For this review, take the finished solid that the model builds, in its own axes (mm). Face numbers are marked on the shaded views. A direction names the side the tool comes from. Coordinates: 2 decimals unless noted, no trailing zeros. Loops run counter-clockwise (first coordinate to the right, second up) from the corner with the lowest first, then second, coordinate; pieces in that order, holes last. Notation, with made-up numbers: M 20,-12 L 44,-12 A21 ccw 44,9 Z; hole C 58.25,61.5 d9. An arc over 180 degrees is marked long. Put each result on its own line as item: value.
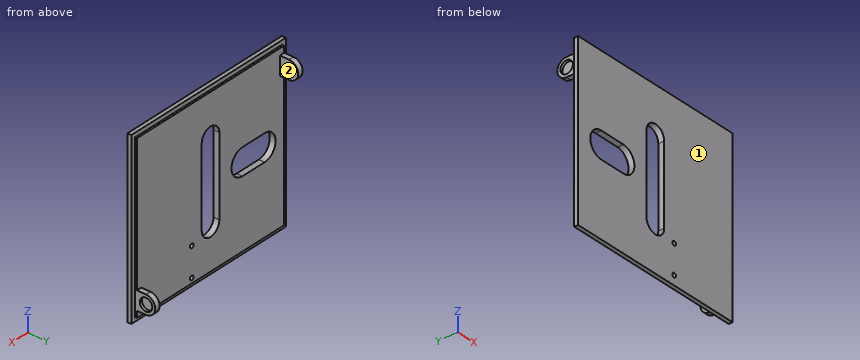
```python
from build123d import *

# Parameters (mm, degrees)
SKETCH1_W                       = 140
SKETCH1_H                       = 130
BOSS_EXTRUDE1_DEPTH             = 3
SKETCH2_W                       = 133.6
SKETCH2_H                       = 123.6
BOSS_EXTRUDE2_DEPTH             = 1.5
SKETCH5_W                       = 4
SKETCH5_H                       = 14
BOSS_EXTRUDE3_DEPTH             = 14
SKETCH6_R                       = 4.775
CUT_EXTRUDE3_DEPTH              = 2
FILLET1_RADIUS                  = 7
FILLET1_LENGTH                  = 4
CIRPATTERN2_COUNT               = 2
FILLET1_OF_CIRPATTERN2_2_RADIUS = 7
FILLET1_OF_CIRPATTERN2_2_LENGTH = 4
CUT_EXTRUDE4_DEPTH              = 97.545326143
CUT_EXTRUDE5_DEPTH              = 98.29979445
SKETCH9_R                       = 1.6
CUT_EXTRUDE6_DEPTH              = 98.29979445


with BuildPart() as part:
    # Sketch1 → Boss-Extrude1 (new body)
    with BuildSketch(Plane(origin=(0, 0, 0), x_dir=(1, 0, 0), z_dir=(0, 1, 0))):
        Rectangle(SKETCH1_W, SKETCH1_H)
    extrude(amount=BOSS_EXTRUDE1_DEPTH)

    # Sketch2 → Boss-Extrude2 (add)
    with BuildSketch(Plane(origin=(0, 3, 0), x_dir=(1, 0, 0), z_dir=(0, 1, 0))):
        Rectangle(SKETCH2_W, SKETCH2_H)
    extrude(amount=BOSS_EXTRUDE2_DEPTH)

    # Sketch5 → Boss-Extrude3 (add)
    with BuildSketch(Plane(origin=(0, 4.5, 0), x_dir=(1, 0, 0), z_dir=(0, 1, 0))):
        with Locations((-64.8, -49.8)):
            Rectangle(SKETCH5_W, SKETCH5_H)
    boss_extrude3 = extrude(amount=BOSS_EXTRUDE3_DEPTH)

    # Sketch6 → Cut-Extrude3 (cut)
    with BuildSketch(Plane.ZY.offset(66.8)):
        with Locations((49.8, 11.5)):
            Circle(SKETCH6_R)
    cut_extrude3 = extrude(amount=-CUT_EXTRUDE3_DEPTH, mode=Mode.SUBTRACT)

    # Fillet1: full round fillet: the end face becomes a half cylinder, R = half its width
    fillet1_face = Plane((-64.8, 18.5, 49.8), x_dir=(1, 0, 0), z_dir=(0, 1, 0))  # on the end face: x along it, z out of the body
    fillet1_slab = fillet1_face.offset(-FILLET1_RADIUS / 2) * Box(FILLET1_LENGTH, 2 * FILLET1_RADIUS, FILLET1_RADIUS, mode=Mode.PRIVATE)  # the body's end, R deep
    fillet1_round = Plane((-64.8, 11.5, 49.8), x_dir=(0, 1, 0), z_dir=(1, 0, 0)) * Cylinder(FILLET1_RADIUS, FILLET1_LENGTH, mode=Mode.PRIVATE)  # its axis R under the face
    add(fillet1_slab - fillet1_round, mode=Mode.SUBTRACT)

    # CirPattern2: Boss-Extrude3, Cut-Extrude3 ×2 about axis
    cirpattern2_axis = Axis((0, 0, 0), (0, 1, 0))
    add([boss_extrude3.rotate(cirpattern2_axis, i * 360 / CIRPATTERN2_COUNT) for i in range(1, CIRPATTERN2_COUNT)])
    add([cut_extrude3.rotate(cirpattern2_axis, i * 360 / CIRPATTERN2_COUNT) for i in range(1, CIRPATTERN2_COUNT)], mode=Mode.SUBTRACT)

    # Fillet1 of CirPattern2 2: full round fillet: the end face becomes a half cylinder, R = half its width
    fillet1_of_cirpattern2_2_face = Plane((64.8, 18.5, -49.8), x_dir=(-1, 0, 0), z_dir=(0, 1, 0))  # on the end face: x along it, z out of the body
    fillet1_of_cirpattern2_2_slab = fillet1_of_cirpattern2_2_face.offset(-FILLET1_OF_CIRPATTERN2_2_RADIUS / 2) * Box(FILLET1_OF_CIRPATTERN2_2_LENGTH, 2 * FILLET1_OF_CIRPATTERN2_2_RADIUS, FILLET1_OF_CIRPATTERN2_2_RADIUS, mode=Mode.PRIVATE)  # the body's end, R deep
    fillet1_of_cirpattern2_2_round = Plane((64.8, 11.5, -49.8), x_dir=(0, 1, 0), z_dir=(-1, 0, 0)) * Cylinder(FILLET1_OF_CIRPATTERN2_2_RADIUS, FILLET1_OF_CIRPATTERN2_2_LENGTH, mode=Mode.PRIVATE)  # its axis R under the face
    add(fillet1_of_cirpattern2_2_slab - fillet1_of_cirpattern2_2_round, mode=Mode.SUBTRACT)

    # Sketch7 → Cut-Extrude4 (cut, through all)
    with BuildSketch(Plane(origin=(0, 4.5, 0), x_dir=(1, 0, 0), z_dir=(0, 1, 0))):
        with BuildLine():
            Line((-8, -30), (-8, 30))
            ThreePointArc((-8, 30), (0, 38), (8, 30))
            Line((8, 30), (8, -30))
            ThreePointArc((8, -30), (0, -38), (-8, -30))
        make_face()
    extrude(amount=-CUT_EXTRUDE4_DEPTH, mode=Mode.SUBTRACT)

    # Sketch8 → Cut-Extrude5 (cut, through all)
    with BuildSketch(Plane.XZ):
        with BuildLine():
            Line((-49, 10), (-29, 10))
            ThreePointArc((-29, 10), (-19, 0), (-29, -10))
            Line((-29, -10), (-49, -10))
            ThreePointArc((-49, -10), (-59, 0), (-49, 10))
        make_face()
    extrude(amount=-CUT_EXTRUDE5_DEPTH, mode=Mode.SUBTRACT)

    # Sketch9 → Cut-Extrude6 (cut, through all)
    with BuildSketch(Plane.XZ):
        with Locations(Location((17, -36, 0), (0, 0, 270))):
            Circle(SKETCH9_R)
        with Locations(Location((17, -58, 0), (0, 0, 270))):
            Circle(SKETCH9_R)
    extrude(amount=-CUT_EXTRUDE6_DEPTH, mode=Mode.SUBTRACT)


solid = part.part
```
(1) For pin 1 (3 mm diameter, centred on x = 65, y = 9.5, fed in from -Z); pin 2 (10 mm diameter, centred on x = 53, z = 8.5, fed in from +Y); pin 3 (11 mm diameter, centred on y = 11.5, z = -49.8, fed in from +X), all flat-tipped, find the tip position at first contact; note any pin that passes through.
Determined:
pin 1: stops at z = -56.8
pin 2: stops at y = 4.5
pin 3: stops at x = 66.8
(2) Add section D-D (z = 51.5). Write out the cut boundary in (x, y).
Determined:
outline: M -70,0 L 70,0 L 70,3 L 66.8,3 L 66.8,4.5 L -62.8,4.5 L -62.8,18.29 L -66.8,18.29 L -66.8,15.96 L -64.8,15.96 L -64.8,7.04 L -66.8,7.04 L -66.8,3 L -70,3 Z
(3) Tool access review of the marked faces 1 and 2: name each direction out of +Z, -Z, +X, -X, +Y, -Y from which nothing blocks a thin tool from reaching the whole face with its end or side.
Determined:
face 1: +Z, -Z, +X, -X, -Y
face 2: +Z, -Z, +X, +Y
(4) Add section B-B (y = 8.5). Write out the cut boundary in (x, z).
Determined:
outline: M -66.8,42.8 L -62.8,42.8 L -62.8,56.8 L -66.8,56.8 L -66.8,53.51 L -64.8,53.51 L -64.8,46.09 L -66.8,46.09 Z; M 62.8,-56.8 L 66.8,-56.8 L 66.8,-53.51 L 64.8,-53.51 L 64.8,-46.09 L 66.8,-46.09 L 66.8,-42.8 L 62.8,-42.8 Z
(5) Add section A-A (z = 0). Write out the cut boundary in (x, y), plus the area to 3 significant figures.
Determined:
outline: M -70,0 L -59,0 L -59,4.5 L -66.8,4.5 L -66.8,3 L -70,3 Z; M -19,0 L -8,0 L -8,4.5 L -19,4.5 Z; M 8,0 L 70,0 L 70,3 L 66.8,3 L 66.8,4.5 L 8,4.5 Z
area: 368 mm^2
(6) Wall thickness on line 1 along X through (y, z) = (1.55, -58); line 2 along Y through (x, z) = (-33, -27); line 3 along Y through (x, z) = (65.75, -49.8) (3 decimals): over which ranges is each line inside the solid? List them lowest first. Write a range as [from, to].
Determined:
line 1: x = [-70, 15.4], [18.6, 70]
line 2: y = [0, 4.5]
line 3: y = [0, 6.725], [16.275, 18.5]
(7) Add section C-C (x = 2). Write out the cut boundary in (y, z), plus the area to 3 significant figures.
Determined:
outline: M 0,-65 L 3,-65 L 3,-61.8 L 4.5,-61.8 L 4.5,-37.75 L 0,-37.75 Z; M 0,37.75 L 4.5,37.75 L 4.5,61.8 L 3,61.8 L 3,65 L 0,65 Z
area: 236 mm^2
